Check sheet for the modelled part. Datum: model origin and axes. Units: mm. Face numbers are marked on the shaded views. A direction names the side the tool comes from. Coordinates: 2 decimals unless noted, no trailing zeros. Loops run counter-clockwise (first coordinate to the right, second up) from the corner with the lowest first, then second, coordinate; pieces in that order, holes last. Notation, with made-up numbers: M 19,44 L 50,44 A13 cw 50,65 Z; hole C 62.25,85.25 d1. An arc over 180 degrees is marked long. Use CSV: the item, a comma, the result in double quotes. Start each with the question number.
(1) Section check B-B on x = 38.1. Record the cut outline in (y, z) (1 decimal), and give its area (3 significant figures).
(2) Scan lines: line 1 (Y direction, x = 38.1, z = 21.75) (3 decimals); line 2 (Y direction, x = -38.1, z = 21.55) (3 decimals); line 3 (X direction, y = -6, z = 11). Record each from-to range of solid material in increasing order.
(3) Section check D-D on y = 0. Record the cut outline in (x, z), and give its area (3 significant figures).
(4) Set-up check for the marked faces 4 and 5: record each of +Z, -Z, +X, -X, +Y, -Y from which the full face is reachable in a straight line by a thin tool's end or side.
(5) Go/stop test with flat-tipped pins: pin 1 Ø7 at (x, y) = (38.1, 17.38) entering from +Z; pin 2 Ø2 at (y, z) = (8, 18) entering from +X; pin 3 Ø6 at (y, z) = (1.5, 5.5) entering from -X; pin 4 Ø5 at (x, z) = (7.5, 8.5) entering from +Y (3 decimals). Record where each tip stops, or that it passes through.
(6) Draft check along Y on the marked faces 1, 2 and 3. Enter one of: pulls with the +Y half, pulls with the -Y half, needs draft (parallel to the pull), parting line crosses it, or undercut.
(7) Section check A-A on z = 21.75. Give the number of separate pieces and of enclosed holes in the cut face, and give its area (3 significant figures).
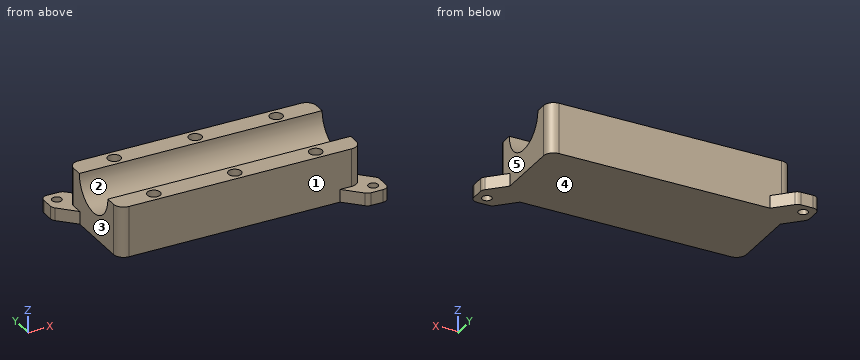
from build123d import *

# Parameters (mm, degrees)
SKETCH1_W               = 114.3
SKETCH1_H               = 44.45
BOSS_EXTRUDE1_DEPTH     = 5
BOSS_EXTRUDE2_DEPTH     = 114.3
SKETCH3_R               = 3.025
CUT_EXTRUDE1_DEPTH      = 5.5
LPATTERN1_COUNT         = 2
LPATTERN1_PITCH         = 38.1
LPATTERN1_COL_COUNT     = 2
LPATTERN1_COL_PITCH     = 38.1
MIRROR1_COPY_1_SKETCH_R = 3.025
MIRROR1_COPY_1_DEPTH    = 5.5
MIRROR1_COPY_2_SKETCH_R = 3.025
MIRROR1_COPY_2_DEPTH    = 5.5
SKETCH4_W               = 10.16
SKETCH4_H               = 10.16
BOSS_EXTRUDE3_DEPTH     = 6
M4_CLEARANCE_HOLE1_D    = 4.5
FILLET3_R               = 3.175
FILLET4_R               = 4.7625


with BuildPart() as part:
    # Sketch1 → Boss-Extrude1 (new body)
    with BuildSketch(Plane.XY):
        Rectangle(SKETCH1_W, SKETCH1_H)
    extrude(amount=BOSS_EXTRUDE1_DEPTH)

    # Sketch2 → Boss-Extrude2 (add)
    with BuildSketch(Plane.ZY.offset(57.15)):
        with BuildLine():
            Line((23.8125, 22.225), (5, 22.225))
            Line((5, 22.225), (5, -22.225))
            Line((5, -22.225), (23.8125, -22.225))
            Line((23.8125, -22.225), (23.8125, -12.5269))
            ThreePointArc((23.8125, -12.5269), (11.2856, 0), (23.8125, 12.5269))
            Line((23.8125, 12.5269), (23.8125, 22.225))
        make_face()
    extrude(amount=-BOSS_EXTRUDE2_DEPTH)

    # Sketch3 → Cut-Extrude1 (cut)
    with BuildSketch(Plane.XY.offset(23.8125)):
        with Locations((0, 17.37595)):
            Circle(SKETCH3_R)
    cut_extrude1 = extrude(amount=-CUT_EXTRUDE1_DEPTH, mode=Mode.SUBTRACT)

    # LPattern1: Cut-Extrude1 ×2
    with Locations(*[(i * LPATTERN1_PITCH, 0, 0) for i in range(1, LPATTERN1_COUNT)]):
        add(cut_extrude1, mode=Mode.SUBTRACT)

    # LPattern1 col: Cut-Extrude1 ×2
    with Locations(*[(-i * LPATTERN1_COL_PITCH, 0, 0) for i in range(1, LPATTERN1_COL_COUNT)]):
        add(cut_extrude1, mode=Mode.SUBTRACT)

    # Mirror1: Cut-Extrude1 across plane
    add(cut_extrude1.mirror(Plane.ZX), mode=Mode.SUBTRACT)

    # Mirror1 copy 1 sketch → Mirror1 copy 1 (cut)
    with BuildSketch(Plane(origin=(38.1, 0, 23.8125), x_dir=(1, 0, 0), z_dir=(0, 0, 1))):
        with Locations((0, -17.37595)):
            Circle(MIRROR1_COPY_1_SKETCH_R)
    extrude(amount=-MIRROR1_COPY_1_DEPTH, mode=Mode.SUBTRACT)

    # Mirror1 copy 2 sketch → Mirror1 copy 2 (cut)
    with BuildSketch(Plane(origin=(-38.1, 0, 23.8125), x_dir=(1, 0, 0), z_dir=(0, 0, 1))):
        with Locations((0, -17.37595)):
            Circle(MIRROR1_COPY_2_SKETCH_R)
    extrude(amount=-MIRROR1_COPY_2_DEPTH, mode=Mode.SUBTRACT)

    # Sketch4 → Boss-Extrude3 (add)
    with BuildSketch(Plane.XY):
        Polygon((-65.7225, 30.7975), (-55.5625, 20.6375), (-65.7225, 20.6375), align=None)
        Polygon((-65.7225, 30.7975), (-55.5625, 30.7975), (-55.5625, 20.6375), align=None)
        with Locations((60.6425, -25.7175)):
            Rectangle(SKETCH4_W, SKETCH4_H)
        Polygon((-55.5625, 30.7975), (-60.6425, 25.7175), (-57.15, 22.225), (-55.5625, 22.225), align=None)
        Polygon((-46.99, 22.225), (-55.5625, 30.7975), (-55.5625, 22.225), align=None)
        Polygon((-60.6425, 25.7175), (-65.7225, 20.6375), (-57.15, 20.6375), (-57.15, 22.225), align=None)
        Polygon((-57.15, 20.6375), (-65.7225, 20.6375), (-57.15, 12.065), align=None)
        Polygon((57.15, -20.6375), (65.7225, -20.6375), (57.15, -12.065), align=None)
        Polygon((46.99, -22.225), (55.5625, -30.7975), (55.5625, -22.225), align=None)
    extrude(amount=BOSS_EXTRUDE3_DEPTH)

    # M4 Clearance Hole1 (through all)
    with Locations(Plane.XY.offset(6)):
        with Locations((-60.6425, 25.7175), (60.6425, -25.7175)):
            Hole(M4_CLEARANCE_HOLE1_D / 2)

    # Fillet3
    fillet3_edges = [part.edges().sort_by_distance(p)[0] for p in [
        (-55.5625, 30.7975, 3),
        (-65.7225, 30.7975, 3),
        (-65.7225, 20.6375, 3),
        (55.5625, -30.7975, 3),
        (65.7225, -30.7975, 3),
        (65.7225, -20.6375, 3),
    ]]
    fillet(fillet3_edges, radius=FILLET3_R)

    # Fillet4
    fillet4_edges = [part.edges().sort_by_distance(p)[0] for p in [
        (57.15, -22.225, 14.90625),
        (-57.15, -22.225, 11.90625),
        (-57.15, 22.225, 14.90625),
        (57.15, 22.225, 11.90625),
    ]]
    fillet(fillet4_edges, radius=FILLET4_R)


solid = part.part
Outcome:
1,outline,"M -22.2,0 L 22.2,0 L 22.2,23.8 L 20.4,23.8 L 20.4,18.3 L 14.4,18.3 L 14.4,23.8 L 12.5,23.8 A12.5 cw -12.5,23.8 L -14.4,23.8 L -14.4,18.3 L -20.4,18.3 L -20.4,23.8 L -22.2,23.8 Z"
1,area,"745 mm²"
2,line 1,"y = -22.225 to -20.401, -14.351 to -12.356, 12.356 to 14.351, 20.401 to 22.225"
2,line 2,"y = -22.225 to -20.401, -14.351 to -12.321, 12.321 to 14.351, 20.401 to 22.225"
2,line 3,"x = -57.15 to 57.15"
3,outline,"M -57.15,0 L 57.15,0 L 57.15,11.29 L -57.15,11.29 Z"
3,area,"1,290 mm²"
4,face 4,"-Z, +X, -X, +Y, -Y"
4,face 5,"+Z, +X, +Y"
5,pin 1,"stops at z = 23.81"
5,pin 2,"passes through"
5,pin 3,"stops at x = -57.15"
5,pin 4,"stops at y = 22.225"
6,face 1,"pulls with the -Y half"
6,face 2,"undercut"
6,face 3,"needs draft"
7,separate pieces,"2"
7,enclosed holes,"6"
7,area,"2,060 mm²"
